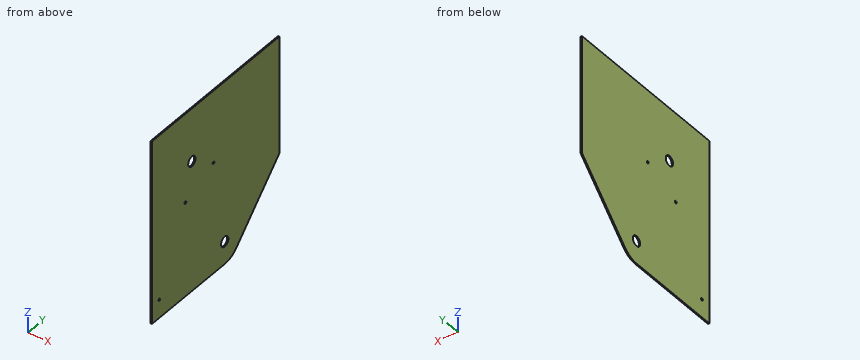
```python
from build123d import *

# Parameters (mm, degrees)
SKETCH1_R           = 12.7
BOSS_EXTRUDE1_DEPTH = 3.175
CUT_EXTRUDE1_REACH  = 5.175
SKETCH2_R           = 3.175
BOSS_EXTRUDE2_DEPTH = 3.175
BOSS_EXTRUDE3_DEPTH = 3.175
CUT_EXTRUDE2_REACH  = 5.175
SKETCH5_R           = 12.7
BOSS_EXTRUDE4_DEPTH = 3.175
SKETCH7_W           = 739.335123301
SKETCH7_H           = 711.050730063
CUT_EXTRUDE3_DEPTH  = 3.175


with BuildPart() as part:
    # Sketch1 → Boss-Extrude1 (new body)
    with BuildSketch(Plane(origin=(0, 0, 0), x_dir=(0, 0, -1), z_dir=(1, 0, 0))):
        with BuildLine():
            Line((-217.899389282, 130.521477737), (17.58316119, 54.3778902))
            ThreePointArc((17.58316119, 54.3778902), (46.211471314, 33.624729277), (57.15, 0))
            Line((57.15, 0), (57.15, -254))
            Line((57.15, -254), (0, -254))
            ThreePointArc((0, -254), (-220.984677461, -125.226883405), (-217.899389282, 130.521477737))
        make_face()
        Circle(SKETCH1_R, mode=Mode.SUBTRACT)
    extrude(amount=BOSS_EXTRUDE1_DEPTH)

    # Sketch2 → Cut-Extrude1 (cut, up to next)
    with BuildSketch(Plane(origin=(3.175, 0, 0), x_dir=(0, 0, -1), z_dir=(1, 0, 0)), mode=Mode.PRIVATE) as cut_extrude1_sk1:
        with Locations((11.103289152, -228.181271676)):
            Circle(SKETCH2_R)
    cut_extrude1_tool1 = extrude(cut_extrude1_sk1.sketch, amount=-CUT_EXTRUDE1_REACH, mode=Mode.PRIVATE) & part.part
    add(cut_extrude1_tool1.solids().sort_by_distance((3.175, -228.181272, -11.103289))[0], mode=Mode.SUBTRACT)
    # Sketch2 → Cut-Extrude1 (cut, up to next)
    with BuildSketch(Plane(origin=(3.175, 0, 0), x_dir=(0, 0, -1), z_dir=(1, 0, 0)), mode=Mode.PRIVATE) as cut_extrude1_sk2:
        with Locations((-180.989788445, -137.156185968)):
            Circle(SKETCH2_R)
    cut_extrude1_tool2 = extrude(cut_extrude1_sk2.sketch, amount=-CUT_EXTRUDE1_REACH, mode=Mode.PRIVATE) & part.part
    add(cut_extrude1_tool2.solids().sort_by_distance((3.175, -137.156186, 180.989788))[0], mode=Mode.SUBTRACT)
    # Sketch2 → Cut-Extrude1 (cut, up to next)
    with BuildSketch(Plane(origin=(3.175, 0, 0), x_dir=(0, 0, -1), z_dir=(1, 0, 0)), mode=Mode.PRIVATE) as cut_extrude1_sk3:
        with Locations((-223.548763187, -39.27724509)):
            Circle(SKETCH2_R)
    cut_extrude1_tool3 = extrude(cut_extrude1_sk3.sketch, amount=-CUT_EXTRUDE1_REACH, mode=Mode.PRIVATE) & part.part
    add(cut_extrude1_tool3.solids().sort_by_distance((3.175, -39.277245, 223.548763))[0], mode=Mode.SUBTRACT)

    # Sketch3 → Boss-Extrude2 (add)
    with BuildSketch(Plane(origin=(3.175, 0, 0), x_dir=(0, 0, -1), z_dir=(1, 0, 0))):
        with BuildLine():
            Line((0, -254), (-254, -254))
            Line((-254, -254), (-254, 0))
            ThreePointArc((-254, 0), (-179.605122421, -179.605122421), (0, -254))
        make_face()
    extrude(amount=-BOSS_EXTRUDE2_DEPTH)

    # Sketch4 → Boss-Extrude3 (add)
    with BuildSketch(Plane(origin=(3.175, 0, 0), x_dir=(0, 0, -1), z_dir=(1, 0, 0))):
        with BuildLine():
            Line((-254, -254), (-406.4, -254))
            Line((-406.4, -254), (-406.4, 191.473394235))
            Line((-406.4, 191.473394235), (-217.899389282, 130.521477737))
            ThreePointArc((-217.899389282, 130.521477737), (-244.808542414, 67.710985528), (-254, 0))
            Line((-254, 0), (-254, -254))
        make_face()
    extrude(amount=-BOSS_EXTRUDE3_DEPTH)

    # Sketch5 → Cut-Extrude2 (cut, up to next)
    with BuildSketch(Plane(origin=(3.175, 0, 0), x_dir=(0, 0, -1), z_dir=(1, 0, 0)), mode=Mode.PRIVATE) as cut_extrude2_sk1:
        with Locations((-272.235522473, -114.629596607)):
            Circle(SKETCH5_R)
    cut_extrude2_tool1 = extrude(cut_extrude2_sk1.sketch, amount=-CUT_EXTRUDE2_REACH, mode=Mode.PRIVATE) & part.part
    add(cut_extrude2_tool1.solids().sort_by_distance((3.175, -114.629597, 272.235522))[0], mode=Mode.SUBTRACT)

    # Sketch6 → Boss-Extrude4 (add)
    with BuildSketch(Plane(origin=(3.175, 0, 0), x_dir=(0, 0, -1), z_dir=(1, 0, 0))):
        with BuildLine():
            Line((40.411152545, 40.411152545), (-406.4, 487.22230509))
            Line((-406.4, 487.22230509), (-406.4, 191.473394235))
            Line((-406.4, 191.473394235), (17.58316119, 54.3778902))
            ThreePointArc((17.58316119, 54.3778902), (29.826205702, 48.749563623), (40.411152545, 40.411152545))
        make_face()
    extrude(amount=-BOSS_EXTRUDE4_DEPTH)

    # Sketch7 → Cut-Extrude3 (cut)
    with BuildSketch(Plane(origin=(3.175, 0, 0), x_dir=(0, 0, -1), z_dir=(1, 0, 0))):
        with Locations((-36.73243835, 546.025365032)):
            Rectangle(SKETCH7_W, SKETCH7_H)
    extrude(amount=-CUT_EXTRUDE3_DEPTH, mode=Mode.SUBTRACT)


solid = part.part
```
Geometry check sheet. Reference: the model listing, model coordinates, mm. Give positions to 0.01 mm unless a question says otherwise; leave off trailing zeros. Write each loop counter-clockwise with the first axis right and the second up, starting at its lowest first coordinate (ties: lowest second). Pieces come first, ordered by that corner, then holes.
1) Section check B-B, the plane x = 2.5. Record the boundary of the cut face in (y, z) (3 decimals).
2) Section check A-A, the plane z = 0. Record the boundary of the cut face in (x, y) (3 decimals), and give its area (3 significant figures).
3) Material ranges on L1, parallel to Y at x = 1.35, z = -9.5; L2, parallel to Z at x = 0.2, y = -5; L3, parallel to Y at x = 2, z = 0, recorded low to high.
4) Section check C-C, the plane y = 61. Record the boundary of the cut face in (x, z) (3 decimals).
5) Gauge pin test, flat end, axial feed: pin 1 (5.5 mm diameter, centred on y = -39.28, z = 223.55, fed in from -X). Record the tip position at first contact, or that the pin passes through.
Computed:
1. outline: (-254, -57.15) - (0, -57.15) arc R57.15 ccw to (40.411, -40.411) - (190.5, 109.678) - (190.5, 406.4) - (-254, 406.4) - close; hole circle Ø6.35 at (-228.181, -11.103); hole circle Ø6.35 at (-137.156, 180.99); hole circle Ø25.4 at (-114.63, 272.236); hole circle Ø6.35 at (-39.277, 223.549); hole circle Ø25.4 at (0, 0)
2. outline: (0, -254) - (3.175, -254) - (3.175, -12.7) - (0, -12.7) - close; (0, 12.7) - (3.175, 12.7) - (3.175, 80.822) - (0, 80.822) - close
2. area: 982 mm2
3. L1: y = -254 to -230.92, -225.44 to -8.43, 8.43 to 71.32
3. L2: z = -57.15 to -11.67, 11.67 to 406.4
3. L3: y = -254 to -12.7, 12.7 to 80.82
4. outline: (0, -19.822) - (3.175, -19.822) - (3.175, 406.4) - (0, 406.4) - close
5. pin 1: passes through
